```python
from build123d import *

# Parameters (mm, degrees)
F0_R     = 10.9
F1_DEPTH = 6.35


# Not quite as in the source:
# - a length typed as a fraction of an inch, garbled in the dataset ("3 / 203.2 mm" for 3/8 in), is restored


with BuildPart() as f1:
    # F0 (on Top) → F1 (new body)
    with BuildSketch(Plane.XY):
        Polygon((12.0834760459, 18.5353325598), (23.2533272356, 35.6692190058), (0, 44.2333527703), (-8.7317753371, 41.5979945749), (-38.6247036873, 32.5759376999), (-18.593203622, 21.0107457448), (-22.0938068874, 1.1969309419), (-42.51711341, 2.3033626056), (-38.3072071936, -22.1166763852), (-34.5838293668, -25.6138377102), (-32.9914432749, -27.1094772381), (-8.8992377565, -49.7379434568), (-8.8992377565, -26.6075595468), (10.0103308414, -19.7322635017), (19.2637861744, -37.9725816114), (38.3072071936, -22.1166763852), (39.4741488289, -17.1435559367), (39.973217609, -15.0166893646), (47.5239414439, 17.162005757), (27.4924413785, 5.5968138019), align=None)
        with Locations((-23.4244655113, -14.9711193807)):
            Circle(F0_R, mode=Mode.SUBTRACT)
        with Locations((24.5570029423, -13.0304875769)):
            Circle(F0_R, mode=Mode.SUBTRACT)
        Circle(F0_R, mode=Mode.SUBTRACT)
        with Locations((-1.0652008007, 27.7795850807)):
            Circle(F0_R, mode=Mode.SUBTRACT)
    extrude(amount=F1_DEPTH)


solid = f1.part
```
Geometry check sheet. Reference: the model listing, model coordinates, mm. A direction names the side the tool comes from. Coordinates: 2 decimals unless noted, no trailing zeros. Order: outer loops, then holes, each group sorted by start corner. A loop starts at its lowest first (then second) coordinate and runs counter-clockwise, first axis right, second up.
Item 1: Tool access check on faces 1 (the flat face through (-8.899, -38, 3)), 2 (the flat face through (19.896, 11.976, 3.131)), 3 (the flat face through (37.65, 11.46, 3.13)). Record the directions out of +Z, -Z, +X, -X, +Y, -Y that give a thin tool (end or side, any length) a straight path to the whole face; none if there is none.
Item 2: Section check C-C (z = 2.75). Enter the section's corners in (x, y), plus the area to 3 significant figures.
Item 3: Section check A-A (y = 12.5). Enter the section's corners in (x, z), plus the area to 3 significant figures.
Item 4: Section check B-B (x = 6). Enter the section's corners in (y, z).
Item 5: Section check D-D (x = 29.5). Enter the section's corners in (y, z).
Item 6: Scan lines: line 1 along X through (y, z) = (7, 3.25); line 2 along Y through (x, z) = (-24, 4.25); line 3 along Y through (x, z) = (-4, 3.75). Record each from-to range of solid material in increasing order.
Item 7: Depth check by flat-ended pin: pin 1 (1.5 mm diameter, centred on y = -33, z = 3, fed in from +X). Enter the tip coordinate at first touch or a pass-through.
Check sheet entries:
1. face 1: +Z, -Z, -Y
1. face 2: +Z, -Z
1. face 3: +Z, -Z, +Y
2. outline: (-42.52, 2.3) - (-38.31, -22.12) - (-8.9, -49.74) - (-8.9, -26.61) - (10.01, -19.73) - (19.26, -37.97) - (38.31, -22.12) - (47.52, 17.16) - (27.49, 5.6) - (12.08, 18.54) - (23.25, 35.67) - (0, 44.23) - (-38.62, 32.58) - (-18.59, 21.01) - (-22.09, 1.2) - close; hole circle Ø21.8 at (-23.42, -14.97); hole circle Ø21.8 at (-1.07, 27.78); hole circle Ø21.8 at (0, 0); hole circle Ø21.8 at (24.56, -13.03)
2. area: 2,970 mm2
3. outline: (-20.1, 0) - (19.27, 0) - (19.27, 6.35) - (-20.1, 6.35) - close; (39.45, 0) - (46.43, 0) - (46.43, 6.35) - (39.45, 6.35) - close
3. area: 294 mm2
4. outline: (-21.19, 0) - (-9.1, 0) - (-9.1, 6.35) - (-21.19, 6.35) - close; (9.1, 0) - (19.48, 0) - (19.48, 6.35) - (9.1, 6.35) - close; (36.08, 0) - (42.02, 0) - (42.02, 6.35) - (36.08, 6.35) - close
5. outline: (-29.45, 0) - (-22.75, 0) - (-22.75, 6.35) - (-29.45, 6.35) - close; (-3.32, 0) - (6.76, 0) - (6.76, 6.35) - (-3.32, 6.35) - close
6. line 1: x = -21.07 to -8.36, 8.36 to 25.82, 29.92 to 45.14
6. line 2: y = -35.55 to -25.86, -4.09 to 1.3, 24.13 to 36.99
6. line 3: y = -24.83 to -10.14, 10.14 to 17.28, 38.28 to 43.03
7. pin 1: stops at x = 26.14
